Build history of the part. All positions in model axes, mm. A direction names the side the tool comes from. Round coordinates to 2 decimals unless told otherwise and drop trailing zeros. Write each loop counter-clockwise with the first axis right and the second up, starting at its lowest first coordinate (ties: lowest second). Pieces come first, ordered by that corner, then holes. Notation, with made-up numbers: (28.5, -16) -> (86.5, -16) arc R22 cw to (86.5, 11) -> close; hole circle Ø1 at (26, 10.25). An arc over 180 degrees is marked (long way). Answer as CSV lines item,"result".
from build123d import *

# Parameters (mm, degrees)
F1_DEPTH = 3.175
F2_DEPTH = 19.05
F3_T     = -2.54


with BuildPart() as f1:
    # F0 (on Top) → F1 (new body)
    with BuildSketch(Plane.XY):
        with BuildLine():
            Line((17.0969952226, -7.4797603572), (-17.0969952226, -7.4797603572))
            ThreePointArc((-17.0969952226, -7.4797603572), (-29.7969952226, -20.1797603572), (-17.0969952226, -32.8797603572))
            Line((-17.0969952226, -32.8797603572), (17.0969952226, -32.8797603572))
            ThreePointArc((17.0969952226, -32.8797603572), (29.7969952226, -20.1797603572), (17.0969952226, -7.4797603572))
        make_face()
    extrude(amount=-F1_DEPTH)

    # F0 (on Top) + F1_face (on face) → F2 (join)
    with BuildSketch(Plane.XY):
        Polygon((127, 57.6001799476), (-127, 57.6001799476), (0, -109.0797603572), align=None)
        with BuildLine():
            ThreePointArc((-17.0969952226, -32.8797603572), (-29.7969952226, -20.1797603572), (-17.0969952226, -7.4797603572))
            Line((-17.0969952226, -7.4797603572), (17.0969952226, -7.4797603572))
            ThreePointArc((17.0969952226, -7.4797603572), (29.7969952226, -20.1797603572), (17.0969952226, -32.8797603572))
            Line((17.0969952226, -32.8797603572), (-17.0969952226, -32.8797603572))
        make_face(mode=Mode.SUBTRACT)
    with BuildSketch(Plane(origin=(0, -20.1797603572, 0), x_dir=(1, 0, 0), z_dir=(0, 0, 1))):
        with BuildLine():
            ThreePointArc((17.0969952226, -12.7), (29.7969952226, 0), (17.0969952226, 12.7))
            Line((17.0969952226, 12.7), (-17.0969952226, 12.7))
            ThreePointArc((-17.0969952226, 12.7), (-29.7969952226, 0), (-17.0969952226, -12.7))
            Line((-17.0969952226, -12.7), (17.0969952226, -12.7))
        make_face()
    extrude(amount=F2_DEPTH)

    # F3
    f3_openings = [f1.faces().sort_by_distance(p)[0] for p in [
        (0, 2.0402, 19.05),
    ]]
    offset(amount=F3_T, openings=f3_openings, kind=Kind.INTERSECTION)


solid = f1.part
1. Cut at D-D, the plane y = -22.5. Write the cut outline in (x, z) (3 decimals).
Results found:
outline,"(-65.969, 0) -> (-29.583, 0) -> (-29.583, -3.175) -> (29.583, -3.175) -> (29.583, 0) -> (65.969, 0) -> (65.969, 19.05) -> (62.775, 19.05) -> (62.775, 2.54) -> (26.989, 2.54) -> (26.989, -0.635) -> (-26.989, -0.635) -> (-26.989, 2.54) -> (-62.775, 2.54) -> (-62.775, 19.05) -> (-65.969, 19.05) -> close"
2. Cut at B-B, the plane x = -93. Write the cut outline in (y, z), then the cut area to 3 significant figures.
Results found:
outline,"(12.98, 0) -> (57.6, 0) -> (57.6, 19.05) -> (55.06, 19.05) -> (55.06, 2.54) -> (17.17, 2.54) -> (17.17, 19.05) -> (12.98, 19.05) -> close"
area,"224 mm2"
3. Which spindle directions (+Z, -Z, +X, -X, +Y, -Y) get a long thin tool onto all of the face, cutting with end or side? Do faces 4 (the flat face through (60.083, -26.034, 10.679)), 5 (the cylindrical face through (29.794, -20.459, -1.565)), 6 (the flat face through (-64.39, -24.57, 9.39)). Say none if no direction does.
Results found:
face 4,"+Z"
face 5,"-Z, +X"
face 6,"+Z, -Z, -X, -Y"
4. Probe line 1 along Z through (x, y) = (-65.5, -23); line 2 along Z through (x, y) = (-17, -27) (3 decimals); line 3 along Y through (x, z) = (9.5, -1.75). List the from-to ranges inside material, lowest first.
Results found:
line 1,"z = 0 to 19.05"
line 2,"z = -3.175 to -0.635"
line 3,"y = -32.88 to -7.48"
5. Mould opens along X. For faces 1 (the flat face through (62.61, -26.91, 9.39)), 2 (the cylindrical face through (-29.794, -19.9, -1.565)), 3 (the flat face through (0, -20, -0.635)) say: +X half, -X half, draft (parallel to the pull), parting line (faces both ways), or undercut.
Results found:
face 1,"+X half"
face 2,"-X half"
face 3,"undercut"
6. Drop flat-ended pins along their axis: pin 1 Ø2 at (x, y) = (93, 19.5) entering from +Z; pin 2 Ø12 at (y, z) = (-78.5, 8.5) entering from -X; pin 3 Ø10 at (y, z) = (-30.5, 7) entering from -X. Give the stop position or say it passes through.
Results found:
pin 1,"stops at z = 2.54"
pin 2,"stops at x = -27.87"
pin 3,"stops at x = -63.68"
7. Cut at A-A, the plane z = 7.25. Write the cut outline in (x, y), then the cut area to 3 significant figures.
Results found:
outline,"(-127, 57.6) -> (0, -109.08) -> (127, 57.6) -> close; hole (-121.87, 55.06) -> (0, -104.89) -> (121.87, 55.06) -> close"
area,"1,680 mm2"
8. Cut at C-C, the plane y = 41. Write the cut outline in (x, z), then the cut area to 3 significant figures.
Results found:
outline,"(-114.35, 0) -> (114.35, 0) -> (114.35, 19.05) -> (111.16, 19.05) -> (111.16, 2.54) -> (-111.16, 2.54) -> (-111.16, 19.05) -> (-114.35, 19.05) -> close"
area,"686 mm2"
